For this review, take the finished solid that the model builds, in its own axes (mm). Face numbers are marked on the shaded views. A direction names the side the tool comes from. Coordinates: 2 decimals unless noted, no trailing zeros. Write each loop counter-clockwise with the first axis right and the second up, starting at its lowest first coordinate (ties: lowest second). Pieces come first, ordered by that corner, then holes. Notation, with made-up numbers: (58.5, 37) - (93.5, 37) arc R6 cw to (93.5, 41) - close; hole circle Ø8 at (77.25, 30). An arc over 180 degrees is marked (long way). Write each question's results on one line, items separated by ' | '.
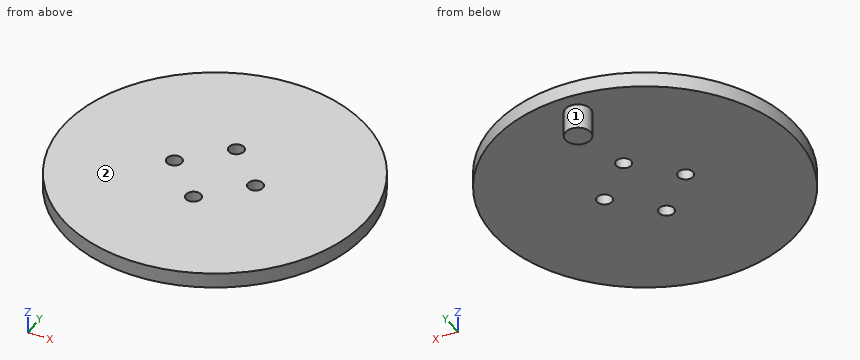
from build123d import *

# Parameters (mm, degrees)
SKETCH3_R           = 30
SKETCH3_R_2         = 1.5
BOSS_EXTRUDE2_DEPTH = 3
SKETCH4_R           = 2.5
BOSS_EXTRUDE3_DEPTH = 5


with BuildPart() as part:
    # Sketch3 → Boss-Extrude2 (new body)
    with BuildSketch(Plane.XY):
        Circle(SKETCH3_R)
        with Locations((-8, 0)):
            Circle(SKETCH3_R_2, mode=Mode.SUBTRACT)
        with Locations((0, 8)):
            Circle(SKETCH3_R_2, mode=Mode.SUBTRACT)
        with Locations((8, 0)):
            Circle(SKETCH3_R_2, mode=Mode.SUBTRACT)
        with Locations((0, -8)):
            Circle(SKETCH3_R_2, mode=Mode.SUBTRACT)
    extrude(amount=BOSS_EXTRUDE2_DEPTH)

    # Sketch4 → Boss-Extrude3 (add)
    with BuildSketch(Plane(origin=(0, 0, 0), x_dir=(-1, 0, 0), z_dir=(0, 0, -1))):
        with Locations((0, 25)):
            Circle(SKETCH4_R)
    extrude(amount=BOSS_EXTRUDE3_DEPTH)


solid = part.part
Q1. Take a section at B-B on z = 1.5. State the section outline as (x, y) points.
Results found:
outline: circle Ø60 at (0, 0); hole circle Ø3 at (-8, 0); hole circle Ø3 at (0, -8); hole circle Ø3 at (0, 8); hole circle Ø3 at (8, 0)
Q2. For pin 1 (10 mm diameter, centred on x = -10, y = 0.5, fed in from -Z); pin 2 (2.5 mm diameter, centred on x = 8, y = 0, fed in from +Z); pin 3 (3 mm diameter, centred on y = -6, z = 1.5, fed in from +X); pin 4 (4 mm diameter, centred on x = -8.5, z = 1.5, fed in from +Y), all flat-tipped, find the tip position at first contact; note any pin that passes through.
Results found:
pin 1: z = 0 | pin 2: through | pin 3: x = 29.66 | pin 4: y = 29.29
Q3. For the marked faces 1 and 2, list the 3-axis set-ups (+Z, -Z, +X, -X, +Y, -Y) from which the entire face can be reached by the end or side of a thin tool; tool diameter is ignored.
Results found:
face 1: -Z | face 2: +Z, +X, -X, +Y, -Y
Q4. Take a section at A-A on x = 0. State the section outline as (y, z) points, plus the area to 3 significant figures.
Results found:
outline: (-30, 0) - (-9.5, 0) - (-9.5, 3) - (-30, 3) - close; (-6.5, 0) - (6.5, 0) - (6.5, 3) - (-6.5, 3) - close; (9.5, 0) - (22.5, 0) - (22.5, -5) - (27.5, -5) - (27.5, 0) - (30, 0) - (30, 3) - (9.5, 3) - close | area: 187 mm2
Q5. Take a section at C-C on x = 8. State the section outline as (y, z) points, plus the area to 3 significant figures.
Results found:
outline: (-28.91, 0) - (-1.5, 0) - (-1.5, 3) - (-28.91, 3) - close; (1.5, 0) - (28.91, 0) - (28.91, 3) - (1.5, 3) - close | area: 164 mm2
Q6. Wall thickness on line 1 along Y through (x, z) = (0, 1.85); line 2 along X through (y, z) = (1, 1.75); line 3 along Z through (x, y) = (12, 8): over which ranges is each line inside the solid? List them lowest first. Write a range as from..to.
Results found:
line 1: -30..-9.5, -6.5..6.5, 9.5..30 | line 2: -29.98..-9.12, -6.88..6.88, 9.12..29.98 | line 3: 0..3
